Verification items for this drawing (mm, ordinates from the low corner). A direction names the side the tool comes from. Round coordinates to 2 decimals unless told otherwise and drop trailing zeros. Loops run counter-clockwise (first coordinate to the right, second up) from the corner with the lowest first, then second, coordinate; pieces in that order, holes last. Notation, with made-up numbers: (-29.75, 70) -> (22.25, 70) arc R37 cw to (22.25, 108) -> close; hole circle Ø1 at (45.5, 51). An arc over 180 degrees is marked (long way). One line per question, with ' | ' between items.
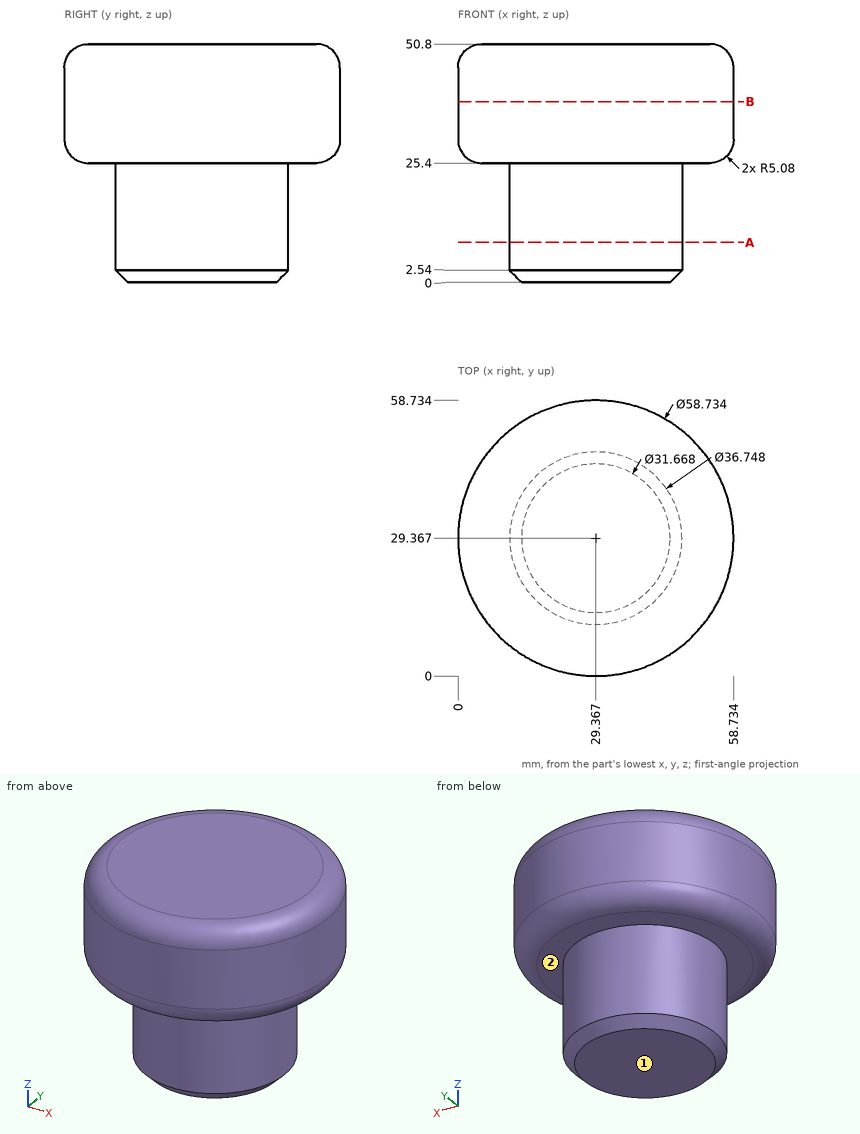
(1) Sectioned sample at B-B, the plane z = 38.5. Record the cut outline in (x, y), and give its area (3 significant figures).
Answer:
outline: circle Ø58.73 at (29.37, 29.37) | area: 2,710 mm2
(2) Go/stop test with flat-tipped pins: pin 1 (8 mm diameter, centred on y = 45.5, z = 15.5, fed in from -X); pin 2 (4 mm diameter, centred on x = 14, z = 26, fed in from -Y); pin 3 (4 mm diameter, centred on x = 18.5, z = 41, fed in from -Y). Record where each tip stops, or that it passes through.
Answer:
pin 1: stops at x = 15.57 | pin 2: stops at y = 4.67 | pin 3: stops at y = 1.37
(3) Scan lines: probe 1 along Z at (x, y) = (49.5, 28.5); probe 2 along Y at (x, z) = (29.5, 6.5); probe 3 along X at (y, z) = (30, 22). Record each from-to range of solid material in increasing order.
Answer:
probe 1: z = 25.4 to 50.8 | probe 2: y = 10.99 to 47.74 | probe 3: x = 11 to 47.73
(4) Set-up check for the marked faces 1 and 2: record each of +Z, -Z, +X, -X, +Y, -Y from which the full face is reachable in a straight line by a thin tool's end or side.
Answer:
face 1: -Z, +X, -X, +Y, -Y | face 2: -Z
(5) Sectioned sample at A-A, the plane z = 8.5. Record the cut outline in (x, y) (1 decimal), and give its area (3 significant figures).
Answer:
outline: circle Ø36.7 at (29.4, 29.4) | area: 1,060 mm2
